Read the model definition and answer for the solid it produces. Units are mm, in the model's axes. Face numbers are marked on the shaded views. A direction names the side the tool comes from. Round coordinates to 2 decimals unless told otherwise and drop trailing zeros. Write each loop counter-clockwise with the first axis right and the second up, starting at its lowest first coordinate (ties: lowest second). Pieces come first, ordered by that corner, then holes. Notation, with made-up numbers: (-31.75, 65) -> (8.25, 65) arc R18 ccw to (8.25, 70) -> close; hole circle Ø2 at (48.25, 33). An arc over 180 degrees is marked (long way). Return JSON: item names as keys, results as strings.
from build123d import *

# Parameters (mm, degrees)
ESQUISSE1_W                     = 36.5
ESQUISSE1_H                     = 7
BOSS_EXTRU_1_DEPTH              = 10
ESQUISSE2_R                     = 5.15
ENL_V_MAT_EXTRU_1_DEPTH         = 10
ESQUISSE3_W                     = 7.9
ESQUISSE3_H                     = 1
ENL_V_MAT_EXTRU_2_DEPTH         = 40
ESQUISSE5_W                     = 36.5
ESQUISSE5_H                     = 7
BOSS_EXTRU_2_DEPTH              = 1.2
ESQUISSE6_R                     = 3.55
ENL_V_MAT_EXTRU_3_DEPTH         = 10
ESQUISSE8_R                     = 2.5
BOSS_EXTRU_3_DEPTH              = 3
R_P_TITION_LIN_AIRE1_COUNT      = 2
R_P_TITION_LIN_AIRE1_PITCH      = 8.2
R_P_TITION_LIN_AIRE1_COUNT_DIR2 = 2
R_P_TITION_LIN_AIRE1_PITCH_DIR2 = 29
R_P_TITION_LIN_AIRE2_COUNT      = 2
R_P_TITION_LIN_AIRE2_PITCH      = 10
ESQUISSE10_R                    = 3.6
ENL_V_MAT_EXTRU_4_DEPTH         = 1.2
ESQUISSE11_W                    = 3.5
ESQUISSE11_H                    = 6.2
ENL_V_MAT_EXTRU_5_DEPTH         = 4
ENL_V_START                     = -2.5
ESQUISSE15_W                    = 3.75
ESQUISSE15_H                    = 2
ENL_V_MAT_EXTRU_7_DEPTH         = 5
ESQUISSE12_W                    = 13.5
ESQUISSE12_H                    = 6.2
ENL_V_MAT_EXTRU_6_DEPTH         = 1
CHANFREIN1_SIZE                 = 1.5


with BuildPart() as part:
    # Esquisse1 → Boss.-Extru.1 (new body)
    with BuildSketch(Plane.XY):
        with Locations((18.25, -3.5)):
            Rectangle(ESQUISSE1_W, ESQUISSE1_H)
    extrude(amount=BOSS_EXTRU_1_DEPTH)

    # Esquisse2 → Enlèv. mat.-Extru.1 (cut)
    with BuildSketch(Plane.XY.offset(10)):
        with Locations((18.25, 0)):
            Circle(ESQUISSE2_R)
    extrude(amount=-ENL_V_MAT_EXTRU_1_DEPTH, mode=Mode.SUBTRACT)

    # Esquisse3 → Enlèv. mat.-Extru.2 (cut)
    with BuildSketch(Plane.ZY):
        with Locations((4.4, -0.5)):
            Rectangle(ESQUISSE3_W, ESQUISSE3_H)
    extrude(amount=-ENL_V_MAT_EXTRU_2_DEPTH, mode=Mode.SUBTRACT)

    # Esquisse5 → Boss.-Extru.2 (add)
    with BuildSketch(Plane(origin=(0, 0, 0), x_dir=(-1, 0, 0), z_dir=(0, 0, -1))):
        with Locations((-18.25, -3.5)):
            Rectangle(ESQUISSE5_W, ESQUISSE5_H)
    boss_extru_2 = extrude(amount=BOSS_EXTRU_2_DEPTH)

    # Esquisse6 → Enlèv. mat.-Extru.3 (cut)
    with BuildSketch(Plane(origin=(0, 0, -1.2), x_dir=(-1, 0, 0), z_dir=(0, 0, -1))):
        with Locations((-18.25, 0)):
            Circle(ESQUISSE6_R)
    extrude(amount=-ENL_V_MAT_EXTRU_3_DEPTH, mode=Mode.SUBTRACT)

    # Esquisse8 → Boss.-Extru.3 (add)
    with BuildSketch(Plane(origin=(0, 0, -1.2), x_dir=(-1, 0, 0), z_dir=(0, 0, -1))):
        with BuildLine():
            Line((-36.5, -7), (-29, -7))
            Line((-29, -7), (-29, -10.5))
            ThreePointArc((-29, -10.5), (-32.75, -14.25), (-36.5, -10.5))
            Line((-36.5, -10.5), (-36.5, -7))
        make_face()
        with Locations((-32.75, -10.5)):
            Circle(ESQUISSE8_R, mode=Mode.SUBTRACT)
    boss_extru_3 = extrude(amount=-BOSS_EXTRU_3_DEPTH)

    # Répétition linéaire1: Boss.-Extru.3 2 × 2
    with Locations(*[(-j * R_P_TITION_LIN_AIRE1_PITCH_DIR2, 0, i * R_P_TITION_LIN_AIRE1_PITCH) for i in range(R_P_TITION_LIN_AIRE1_COUNT) for j in range(R_P_TITION_LIN_AIRE1_COUNT_DIR2) if (i, j) != (0, 0)]):
        add(boss_extru_3)

    # Répétition linéaire2: Boss.-Extru.2 ×2
    with Locations(*[(0, 0, i * R_P_TITION_LIN_AIRE2_PITCH) for i in range(1, R_P_TITION_LIN_AIRE2_COUNT)]):
        add(boss_extru_2)

    # Esquisse10 → Enlèv. mat.-Extru.4 (cut)
    with BuildSketch(Plane.XY.offset(10)):
        with Locations((18.25, 0)):
            Circle(ESQUISSE10_R)
    extrude(amount=-ENL_V_MAT_EXTRU_4_DEPTH, mode=Mode.SUBTRACT)

    # Esquisse11 → Enlèv. mat.-Extru.5 (cut)
    with BuildSketch(Plane.XZ.offset(7)):
        with Locations((9.75, 4.4)):
            Rectangle(ESQUISSE11_W, ESQUISSE11_H)
        with Locations((26.75, 4.4)):
            Rectangle(ESQUISSE11_W, ESQUISSE11_H)
    extrude(amount=-ENL_V_MAT_EXTRU_5_DEPTH, mode=Mode.SUBTRACT)

    # Esquisse15 → Enlèv. mat.-Extru.7 (cut)
    with BuildSketch(Plane(origin=(0, 0, -1.2), x_dir=(-1, 0, 0), z_dir=(0, 0, -1)).offset(ENL_V_START)):
        with Locations((-6.125, -4)):
            Rectangle(ESQUISSE15_W, ESQUISSE15_H)
        with Locations((-30.375, -4)):
            Rectangle(ESQUISSE15_W, ESQUISSE15_H)
    extrude(amount=-ENL_V_MAT_EXTRU_7_DEPTH, mode=Mode.SUBTRACT)

    # Esquisse12 → Enlèv. mat.-Extru.6 (cut)
    with BuildSketch(Plane(origin=(0, -7, 0), x_dir=(-1, 0, 0), z_dir=(0, -1, 0))):
        with Locations((-18.25, -4.4)):
            Rectangle(ESQUISSE12_W, ESQUISSE12_H)
    extrude(amount=-ENL_V_MAT_EXTRU_6_DEPTH, mode=Mode.SUBTRACT)

    # Chanfrein1
    chanfrein1_edges = [part.edges().sort_by_distance(p)[0] for p in [
        (8, -5, 3.8),
        (28.5, -5, 3.8),
        (11.5, -6, 4.4),
        (25, -6, 4.4),
    ]]
    chamfer(chanfrein1_edges, length=CHANFREIN1_SIZE)


solid = part.part
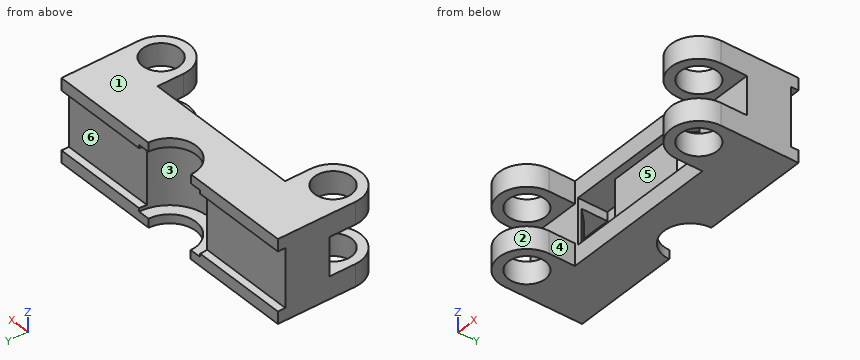
Item 1: Section D-D (x = 18.25) is taken. Give the vertices of the cut face in (y, z), then the cut area to 3 significant figures.
Worked answers:
{"outline": "(-7, -1.2) -> (-3.55, -1.2) -> (-3.55, 0) -> (-5.15, 0) -> (-5.15, 8.8) -> (-3.6, 8.8) -> (-3.6, 10) -> (-7, 10) -> (-7, 7.5) -> (-6, 7.5) -> (-6, 1.3) -> (-7, 1.3) -> close", "area": "18.3 mm2"}
Item 2: Flat-ended cylindrical pins translate along their axes: pin 1 (3.5 mm diameter, centred on x = 31, y = -9.5, fed in from +Z); pin 2 (1.9 mm diameter, centred on x = 9.5, z = 4, fed in from -Y); pin 3 (1 mm diameter, centred on x = 19, z = 0, fed in from -Y). Find the tip coordinate at first contact, or state that the pin passes through.
Worked answers:
{"pin 1": "stops at z = 10", "pin 2": "stops at y = -3", "pin 3": "stops at y = -7"}
Item 3: Section C-C (z = 3) is taken. Give the vertices of the cut face in (x, y).
Worked answers:
{"outline": "(0, -7) -> (8, -7) -> (8, -6.5) -> (6.5, -5) -> (4.25, -5) -> (4.25, -3) -> (11.5, -3) -> (11.5, -4.5) -> (13, -6) -> (23.5, -6) -> (25, -4.5) -> (25, -3) -> (32.25, -3) -> (32.25, -5) -> (30, -5) -> (28.5, -6.5) -> (28.5, -7) -> (36.5, -7) -> (36.5, -1) -> (23.3, -1) arc R5.15 cw to (13.2, -1) -> (0, -1) -> close"}
Item 4: Section A-A (x = 32.75) is taken. Give the vertices of the cut face in (y, z).
Worked answers:
{"outline": "(-14.25, -1.2) -> (-13, -1.2) -> (-13, 1.8) -> (-14.25, 1.8) -> close; (-14.25, 7) -> (-13, 7) -> (-13, 10) -> (-14.25, 10) -> close; (-8, -1.2) -> (0, -1.2) -> (0, 0.45) -> (-1, 0.45) -> (-1, 8.35) -> (0, 8.35) -> (0, 10) -> (-8, 10) -> (-8, 7) -> (-7, 7) -> (-7, 1.8) -> (-8, 1.8) -> close"}
Item 5: Section B-B (y = -11) is taken. State how many separate pieces and enclosed holes the cut face has, then the cut area to 3 significant figures.
Worked answers:
{"separate pieces": "8", "enclosed holes": "0", "area": "30.4 mm2"}
Item 6: For a pull along Z with two mould halves and no side action, classify the marked faces 1, 2 and 3 as released by +Z, released by -Z, zero draft, split by the parting line, or undercut.
Worked answers:
{"face 1": "released by +Z", "face 2": "zero draft", "face 3": "undercut"}
Item 7: A tool of negligible diameter and unlimited length cuts with its end or side. For the marked faces 4, 5 and 6, from which of +Z, -Z, +X, -X, +Y, -Y can it reach the whole face along a straight path? Write none if from no direction.
Worked answers:
{"face 4": "+Z, -Z, -Y", "face 5": "-Y", "face 6": "+X, -X, +Y"}
Item 8: Straight lines are drawn through the part: L1, parallel to Y at x = 32.75, z = 0.75; L2, parallel to Z at x = 5, y = -3.5; L3, parallel to Z at x = 9.5, y = -5. For each, find the intervals that lie inside material, in ascending order. Write a range as [from, to].
Worked answers:
{"L1": "y = [-14.25, -13], [-8, -1]", "L2": "z = [-1.2, 1.3], [6.3, 10]", "L3": "z = [-1.2, 1.3], [7.5, 10]"}
